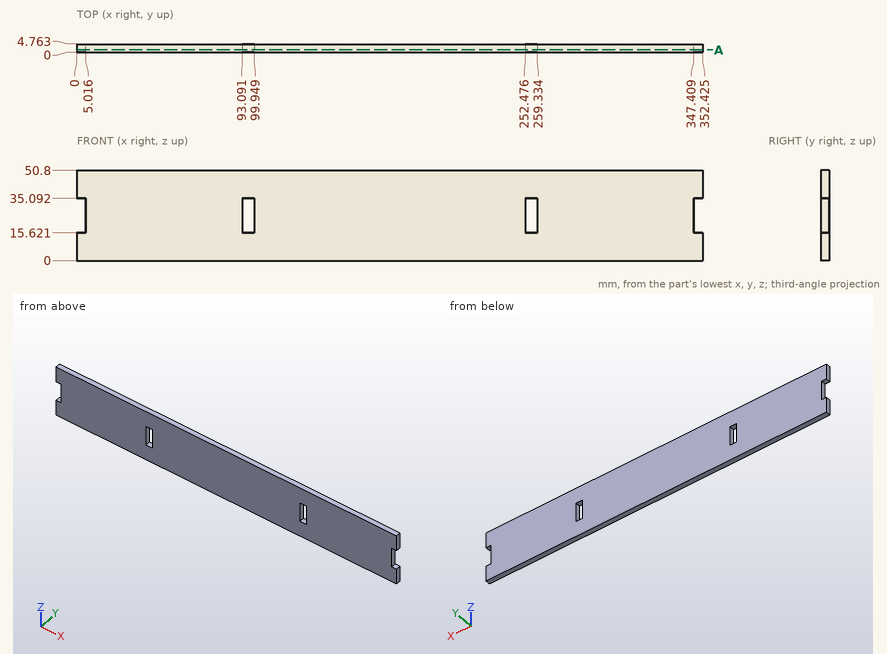
Source: three-view drawing plus pictorial views. Frame: mm from the lowest corner of the part. Give positions to 0.01 mm unless a question says otherwise; leave off trailing zeros. Put each result on its own line as item: value.
Item 1: Section query A-A, the plane y = 1.4. Count the separate pieces of the cut face and the enclosed holes in it, then the cut area to 3 significant figures.
Found:
separate pieces: 1
enclosed holes: 2
area: 17,400 mm^2
Item 2: Contact query for flat-ended pins moving along their axis: pin 1 (2.5 mm diameter, centred on y = 1.5, z = 30, fed in from -X); pin 2 (1 mm diameter, centred on y = 1, z = 12, fed in from -X); pin 3 (2.5 mm diameter, centred on y = 3, z = 24.5, fed in from +X). Output: stop coordinate, or through.
Found:
pin 1: stops at x = 5.02
pin 2: stops at x = 0
pin 3: stops at x = 347.41
Item 3: Ray query, L1, parallel to Z at x = 253.5, y = 2.45. Return the intervals inside material, ascending. Write a range as from..to.
Found:
L1: z = 0..15.62, 35.09..50.8
